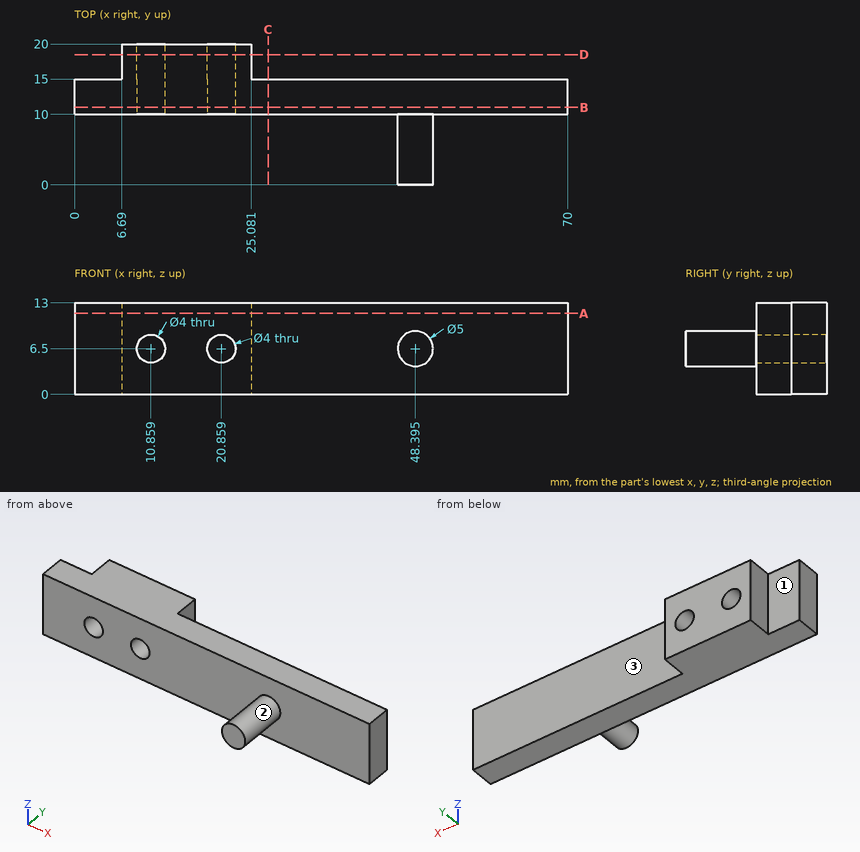
Can you work these out from the drawing? Everything is in mm from the part's minimum corner. A direction names the side the tool comes from. Coordinates: 2 decimals unless noted, no trailing zeros. Loops run counter-clockwise (first coordinate to the right, second up) from the corner with the lowest first, then second, coordinate; pieces in that order, holes last. Notation, with made-up numbers: M -25,-27.75 L 3,-27.75 A22 cw 3,-2.75 Z; hole C -3,2.25 d3. An arc over 180 degrees is marked long. Put each result on its own line as item: value. Start each with the question number.
(1) Will these pins go through, and if not, where does the flat tip stop? P1, Ø4, axis at x = 41.5, z = 8.5, coming from the -Y side; P2, Ø4, axis at x = 42.5, z = 7.5, coming from the +Y side; P3, Ø3, axis at x = 51, y = 4.5, coming from the -Z side.
(2) For the marked faces 1, 2 and 3, which set-ups out of +Z, -Z, +X, -X, +Y, -Y let a thin tool reach every point of the face, with its end or its side?
(3) Suppose I cut it at C-C on x = 27.5. Please give me the cut outline in (y, z).
(4) I need wall thicknesses on line 1 (X direction, y = 15.5, z = 6.5); line 2 (X direction, y = 14.25, z = 6.5); line 3 (Y direction, x = 51, z = 12). Which ranges of each line are inside material? Lowest first, please. Write a range as from..to.
(5) Suppose I cut it at B-B on y = 11. Please give me the cut outline in (x, z).
(6) Suppose I cut it at D-D on y = 18.5. Please give me the cut outline in (x, z).
(7) Suppose I cut it at A-A on z = 11.5. Please give me the cut outline in (x, y), then the cut area to 3 significant figures.
Solutions:
1. P1: stops at y = 10
1. P2: stops at y = 15
1. P3: stops at z = 4.26
2. face 1: +Z, -Z, -X, +Y
2. face 2: -Y
2. face 3: +Z, -Z, +X, +Y
3. outline: M 10,0 L 15,0 L 15,13 L 10,13 Z
4. line 1: x = 6.69..8.86, 12.86..18.86, 22.86..25.08
4. line 2: x = 0..8.86, 12.86..18.86, 22.86..70
4. line 3: y = 10..15
5. outline: M 0,0 L 70,0 L 70,13 L 0,13 Z; hole C 10.86,6.5 d4; hole C 20.86,6.5 d4
6. outline: M 6.69,0 L 25.08,0 L 25.08,13 L 6.69,13 Z; hole C 10.86,6.5 d4; hole C 20.86,6.5 d4
7. outline: M 0,10 L 70,10 L 70,15 L 25.08,15 L 25.08,20 L 6.69,20 L 6.69,15 L 0,15 Z
7. area: 442 mm2
